from build123d import *

# Parameters (mm, degrees)
SKETCH1_W           = 25
SKETCH1_H           = 40
SKETCH1_W_2         = 35
SKETCH1_H_2         = 20
BOSS_EXTRUDE1_DEPTH = 3
SKETCH4_R           = 2.75
CUT_EXTRUDE1_DEPTH  = 3


with BuildPart() as part:
    # Sketch1 → Boss-Extrude1 (new body)
    with BuildSketch(Plane(origin=(0, 0, 0), x_dir=(1, 0, 0), z_dir=(0, 1, 0))):
        with Locations((12.5, -20)):
            Rectangle(SKETCH1_W, SKETCH1_H)
        with Locations((42.5, -30)):
            Rectangle(SKETCH1_W_2, SKETCH1_H_2)
    extrude(amount=BOSS_EXTRUDE1_DEPTH)

    # Sketch4 → Cut-Extrude1 (cut)
    with BuildSketch(Plane(origin=(0, 3, 0), x_dir=(1, 0, 0), z_dir=(0, 1, 0))):
        with Locations((12.5, -10)):
            Circle(SKETCH4_R)
        with Locations((12.5, -30)):
            Circle(SKETCH4_R)
        with Locations((50, -30)):
            Circle(SKETCH4_R)
    extrude(amount=-CUT_EXTRUDE1_DEPTH, mode=Mode.SUBTRACT)


solid = part.part
Model file for the job. Use its own axes, mm. A direction names the side the tool comes from. Coordinates: 2 decimals unless noted, no trailing zeros. Loops run counter-clockwise (first coordinate to the right, second up) from the corner with the lowest first, then second, coordinate; pieces in that order, holes last. Notation, with made-up numbers: (47, 42.5) -> (75, 42.5) arc R15 cw to (75, 60.5) -> close; hole circle Ø8 at (-14, -28). An arc over 180 degrees is marked (long way). Use one line per item in the form item = value. Start each with the question number.
(1) Tool access for faces 5 (the flat face through (0, 1, 20)), 6 (the flat face through (42, 1, 20)): list every direction of +Z, -Z, +X, -X, +Y, -Y with a clear straight run to the whole face (end or side of a thin tool).
(2) Cut at A-A on z = 30. Give the cut face in (x, y).
(3) Pull direction Z, two halves, no side cores. Call faces 1 (the flat face through (12, 1, 0)), 2 (the cylindrical face through (12.142, 1.521, 27.273)), 3 (the cylindrical face through (47.253, 1.521, 29.879)), 4 (the flat face through (60, 1, 30)): pulls with the +Z half, pulls with the -Z half, needs draft (parallel to the pull), parting line crosses it, or undercut.
(4) Cut at B-B on x = 12.5. Give the cut face in (y, z), and give its area (3 significant figures).
(5) Flat gauge pins, fed straight in: pin 1 (9 mm diameter, centred on x = 12.5, z = 10, fed in from -Y); pin 2 (1.5 mm diameter, centred on y = 1.5, z = 12.5, fed in from +X); pin 3 (5 mm diameter, centred on x = 50, z = 30, fed in from +Y). Where does each tip first touch, or does it go through?
(6) Cut at D-D on z = 10. Give the cut face in (x, y).
(7) Probe probe 1 along Z at (x, y) = (12.5, 1.55); probe 2 along X at (y, z) = (2, 30); probe 3 along X at (y, z) = (1.8, 29). List the from-to ranges inside material, lowest first. Write a range as from..to.
(8) Cut at C-C on y = 0.95. Give the cut face in (x, z), and give its area (3 significant figures).
Values:
q1.face_5 = +Z, -Z, -X, +Y, -Y
q1.face_6 = -Z, +X, +Y, -Y
q2.outline = (0, 0) -> (9.75, 0) -> (9.75, 3) -> (0, 3) -> close; (15.25, 0) -> (47.25, 0) -> (47.25, 3) -> (15.25, 3) -> close; (52.75, 0) -> (60, 0) -> (60, 3) -> (52.75, 3) -> close
q3.face_1 = pulls with the -Z half
q3.face_2 = undercut
q3.face_3 = undercut
q3.face_4 = needs draft
q4.outline = (0, 0) -> (3, 0) -> (3, 7.25) -> (0, 7.25) -> close; (0, 12.75) -> (3, 12.75) -> (3, 27.25) -> (0, 27.25) -> close; (0, 32.75) -> (3, 32.75) -> (3, 40) -> (0, 40) -> close
q4.area = 87.0 mm2
q5.pin_1 = 0
q5.pin_2 = 25
q5.pin_3 = through
q6.outline = (0, 0) -> (9.75, 0) -> (9.75, 3) -> (0, 3) -> close; (15.25, 0) -> (25, 0) -> (25, 3) -> (15.25, 3) -> close
q7.probe_1 = 0..7.25, 12.75..27.25, 32.75..40
q7.probe_2 = 0..9.75, 15.25..47.25, 52.75..60
q7.probe_3 = 0..9.94, 15.06..47.44, 52.56..60
q8.outline = (0, 0) -> (25, 0) -> (25, 20) -> (60, 20) -> (60, 40) -> (0, 40) -> close; hole circle Ø5.5 at (12.5, 10); hole circle Ø5.5 at (12.5, 30); hole circle Ø5.5 at (50, 30)
q8.area = 1,630 mm2
